Geometry: final body of the model. Coordinates: model frame, mm. A direction names the side the tool comes from. Coordinates: 2 decimals unless noted, no trailing zeros. Order: outer loops, then holes, each group sorted by start corner. A loop starts at its lowest first (then second) coordinate and runs counter-clockwise, first axis right, second up. Notation, with made-up numbers: (73, 82) -> (77, 82) arc R5 ccw to (77, 86) -> close; hole circle Ø6 at (61.5, -23.5). An arc over 180 degrees is marked (long way). Use CSV: the item, a comma, the result in double quotes. Start each with the question number.
from build123d import *

# Parameters (mm, degrees)
F1_R        = 24.0785224066
F2_DEPTH    = 38.1
F3_DEPTH    = 10.16
F4_W        = 72.8784613311
F4_H        = 14.0676931478
F5_DEPTH    = 38.1
F6_DEPTH    = 0.508
F7_T4_DEPTH = 321.0752082512


# Not quite as in the source:
# - a fillet or chamfer that OpenCascade refuses, or shapes differently, is made with other operations: its cross-section is extruded or revolved along the edge and cut away or added


with BuildPart() as f2:
    # F1 (on face) → F2 (new body)
    with BuildSketch(Plane.XY):
        with BuildLine():
            ThreePointArc((21.3381504126, 25.1467317917), (11.0402076987, 0), (21.3381504126, -25.1467317917))
            ThreePointArc((21.3381504126, -25.1467317917), (60.4791188031, -33.1778787511), (82.7444076987, 0))
            ThreePointArc((82.7444076987, 0), (60.4791188031, 33.1778787511), (21.3381504126, 25.1467317917))
        make_face()
        with Locations((46.6475896537, 0)):
            Circle(F1_R, mode=Mode.SUBTRACT)
    extrude(amount=F2_DEPTH)

    # F0 (on Top) → F3 (join)
    with BuildSketch(Plane.XY):
        with BuildLine():
            ThreePointArc((21.3381504126, -25.1467317917), (11.0402076987, 0), (21.3381504126, 25.1467317917))
            Line((21.3381504126, 25.1467317917), (-70.9246173501, 25.1467317917))
            Line((-70.9246173501, 25.1467317917), (-70.9246173501, -25.1914039254))
            Line((-70.9246173501, -25.1914039254), (21.3381504126, -25.1914039254))
            Line((21.3381504126, -25.1914039254), (21.3381504126, -25.1467317917))
        make_face()
    extrude(amount=F3_DEPTH)

    # F4 (on Top) → F5 (join)
    with BuildSketch(Plane.XY):
        with Locations((-12.2608747333, 0.0976922456)):
            Rectangle(F4_W, F4_H)
    extrude(amount=F5_DEPTH)

    # F6 (cut): a face of the model
    f6_faces = [f2.faces().sort_by_distance(p)[0] for p in [
        (24.1783559322, 0.0976922456, 19.05),
    ]]
    extrude(f6_faces, amount=-F6_DEPTH, mode=Mode.SUBTRACT)

    # F7: chamfer of 59.69 on 1 edges, made by hand


with BuildPart() as f7_tool2:
    # F7_s3 → F7_t4 (new body)
    with BuildSketch(Plane.XZ.offset(-160.6352963712)):
        Polygon((10.9898946011, 38.1), (-48.7001053989, -21.59), (-48.7001053989, 38.1), align=None)
    extrude(amount=F7_T4_DEPTH)

    split(bisect_by=Plane.XY.offset(10.16), keep=Keep.TOP)


with BuildPart() as f2_1:
    add(f2.part)

    # F7_t1: cut F7_tool2
    add(f7_tool2.part, mode=Mode.SUBTRACT)


solid = f2_1.part
(1) Line query: line 1 (Y direction, x = -35.5, z = 3); line 2 (X direction, y = -17.5, z = 11); line 3 (X direction, y = 10, z = 5). Output: solid intervals per line, ascending. Write a range as from..to.
(2) First-contact query: pin 1 (10 mm diameter, centred on x = -2.5, z = 15.5, fed in from +Y); pin 2 (12 mm diameter, centred on x = 10, z = 6.5, fed in from +Y); pin 3 (4 mm diameter, centred on x = 39, z = 12, fed in from -Y). Flat tips, straight axial feed; report the tip coordinate or a pass-through.
(3) Section A-A (y = 0). Return loops of the section in (x, z), then the cut area to 3 significant figures.
(4) Section B-B (x = 51). Return loops of the section in (y, z), then the cut area to 3 significant figures.
(5) Access query for faces 4 (the face through (-24, 25.147, 5)), 5 (the face through (-36, 0, 10.16)), 6 (the face through (-25, -25.191, 5)). Directions: +Z, -Z, +X, -X, +Y, -Y. A direction counts if a zero-diameter tool reaches every point of the face in a straight line with its end or side. Return the directions, or none.
(6) Mould query, pull axis Y, two halves, no side actions, for faces 1 (the face through (0, 7.132, 21)), 2 (the face through (70.7, -1.1, 18.8)), 3 (the face through (54.3, -23.4, 38.1)). Classes: pulls with the +Y half, pulls with the -Y half, needs draft (parallel to the pull), parting line crosses it, or undercut.
(7) Section D-D (x = -12.5). Return loops of the section in (y, z), then the cut area to 3 significant figures.
Check sheet entries:
1,line 1,"y = -25.19..25.15"
1,line 2,"x = 15.6..30.11, 63.19..78.18"
1,line 3,"x = -70.92..24.74, 68.55..81.32"
2,pin 1,"stops at y = 7.13"
2,pin 2,"stops at y = 25.15"
2,pin 3,"stops at y = -35.36"
3,outline,"(-70.92, 0) -> (23.67, 0) -> (23.67, 38.1) -> (10.99, 38.1) -> (-16.95, 10.16) -> (-70.92, 10.16) -> close; (70.73, 0) -> (82.74, 0) -> (82.74, 38.1) -> (70.73, 38.1) -> close"
3,area,"2,160 mm^2"
4,outline,"(-35.62, 0) -> (-23.68, 0) -> (-23.68, 38.1) -> (-35.62, 38.1) -> close; (23.68, 0) -> (35.62, 0) -> (35.62, 38.1) -> (23.68, 38.1) -> close"
4,area,"909 mm^2"
5,face 4,"+Z, -Z, -X, +Y"
5,face 5,"+Z, -X"
5,face 6,"+Z, -Z, -X, -Y"
6,face 1,"pulls with the +Y half"
6,face 2,"undercut"
6,face 3,"needs draft"
7,outline,"(-25.19, 0) -> (25.15, 0) -> (25.15, 10.16) -> (7.13, 10.16) -> (7.13, 14.61) -> (-6.94, 14.61) -> (-6.94, 10.16) -> (-25.19, 10.16) -> close"
7,area,"574 mm^2"
